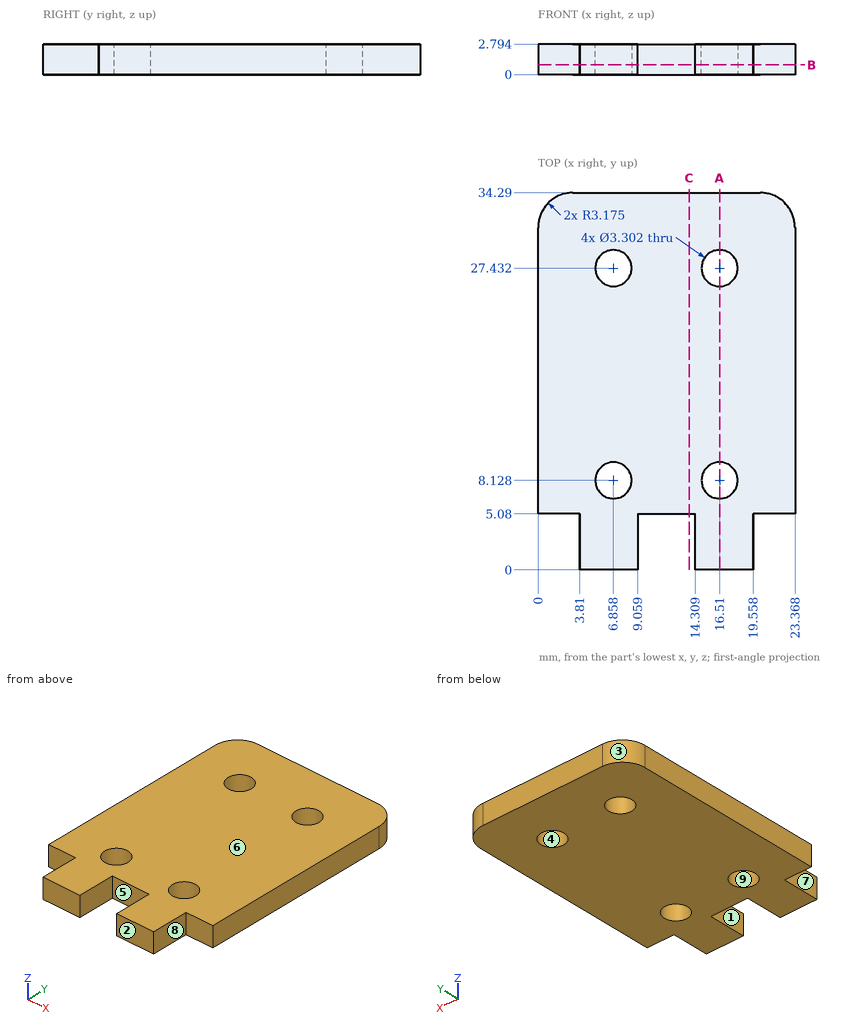
Answer from the drawing. Dimensions are ordinates in mm from the lowest x, y and z of the part. A direction names the side the tool comes from. Round coordinates to 2 decimals unless told otherwise and drop trailing zeros. Loops run counter-clockwise (first coordinate to the right, second up) from the corner with the lowest first, then second, coordinate; pieces in that order, holes last.
(1) Each of these flat-tipped pins is pushed along its axis until it touches: P1, Ø1.4, axis at y = 2.5, z = 2, coming from the +X side; P2, Ø1.4, axis at x = 21.5, z = 1.5, coming from the -Y side; P3, Ø2, axis at x = 16.51, y = 27.432, coming from the -Z side; P4, Ø0.8, axis at y = 3, z = 1, coming from the -X side. Where does it stop, or does it pass through?
Computed values:
P1: stops at x = 19.56
P2: stops at y = 5.08
P3: passes through
P4: stops at x = 3.81
(2) For the marked faces 5, 6, 7, 8 and 9, determine the directions among +Z, -Z, +X, -X, +Y, -Y from which every point of the face is accessible in a straight line to the end or side of a thin tool.
Computed values:
face 5: +Z, -Z, -Y
face 6: +Z, +X, -X, +Y, -Y
face 7: +Z, -Z, -X, -Y
face 8: +Z, -Z, +X, -Y
face 9: +Z, -Z
(3) The part is cut by section C-C, the plane x = 13.75. Give the vertices of the cut face in (y, z).
Computed values:
outline: (5.08, 0) - (34.29, 0) - (34.29, 2.79) - (5.08, 2.79) - close
(4) The part is cut by section B-B, the plane z = 0.9. Give the number of separate pieces and of enclosed holes in the cut face, and give its area (3 significant figures).
Computed values:
separate pieces: 1
enclosed holes: 4
area: 697 mm2
(5) The mould has two halves that part along Y. Classify the marked faces 1, 2, 3 and 4: pulls with the +Y half, pulls with the -Y half, needs draft (parallel to the pull), parting line crosses it, or undercut.
Computed values:
face 1: needs draft
face 2: pulls with the -Y half
face 3: pulls with the +Y half
face 4: undercut
(6) The part is cut by section A-A, the plane x = 16.51. Give the vertices of the cut face in (y, z).
Computed values:
outline: (0, 0) - (6.48, 0) - (6.48, 2.79) - (0, 2.79) - close; (9.78, 0) - (25.78, 0) - (25.78, 2.79) - (9.78, 2.79) - close; (29.08, 0) - (34.29, 0) - (34.29, 2.79) - (29.08, 2.79) - close
(7) Find the intervals of material crossed by L1, parallel to Y at x = 16.51, z = 1.95; L2, parallel to Y at x = 6, z = 0.7; L3, parallel to X at y = 27, z = 0.8 (1 decimal), in increasing order.
Computed values:
L1: y = 0 to 6.48, 9.78 to 25.78, 29.08 to 34.29
L2: y = 0 to 6.72, 9.54 to 26.02, 28.84 to 34.29
L3: x = 0 to 5.3, 8.5 to 14.9, 18.1 to 23.4
